Can you work these out from the drawing? Everything is in mm from the part's minimum corner. A direction names the side the tool comes from. Round coordinates to 2 decimals unless told otherwise and drop trailing zeros. Write each loop counter-clockwise with the first axis right and the second up, starting at its lowest first coordinate (ties: lowest second). Pieces come first, ordered by that corner, then holes. Notation, with made-up numbers: (-27.75, -34.5) - (-12.75, -34.5) arc R35 ccw to (-12.75, 1.5) - close; hole circle Ø2 at (21.5, 61). An arc over 180 degrees is marked (long way). Write each question's results on one line, items separated by ' | '. Start each with the question number.
(1) Please list where these lines run through material, in increasing order: line 1 (Z direction, x = 1.75, y = 4.25); line 2 (X direction, y = 4.25, z = 1.25); line 3 (Y direction, x = 19, z = 19). Write a range as [from, to].
(2) Imagine slicing it at B-B on x = 11.25. Write out the boundary of the cut face in (y, z), then the cut area to 3 significant figures.
(3) Imagine slicing it at A-A on y = 7. Write out the boundary of the cut face in (x, z) (1 decimal).
(4) Imagine slicing it at C-C on z = 12.5. Write out the boundary of the cut face in (x, y).
(5) For P1, Ø4, axis at y = 9, z = 11, coming from the -X side; P2, Ø5, axis at x = 2.5, z = 19, coming from the -Y side; P3, Ø0.9, axis at x = 14.5, z = 24, coming from the +Y side; P4, Ø9.5, axis at x = 12.5, z = 11, coming from the +Y side, each with a flat end and sliding along its axis, tell me the tip position at first contact or that it passes through.
(6) On a 3-axis mill with a long thin cutter (end or side, diameter ignored), from which of +Z, -Z, +X, -X, +Y, -Y can I reach the whole of each face in a straight line? I mean the marked faces 1, 2 and 3. Say none if no direction works.
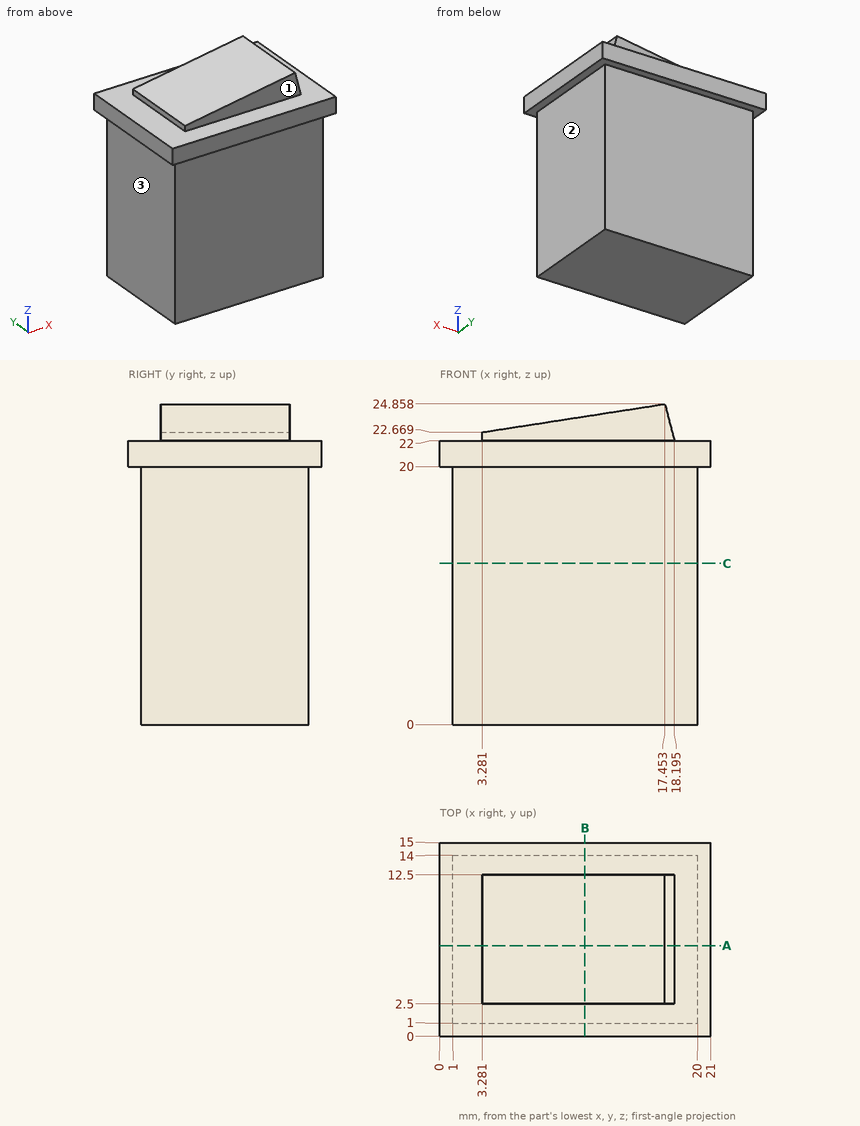
Response:
1) line 1: [0, 22] | line 2: [1, 20] | line 3: [1, 14]
2) outline: (0, 20) - (1, 20) - (1, 0) - (14, 0) - (14, 20) - (15, 20) - (15, 22) - (12.5, 22) - (12.5, 23.9) - (2.5, 23.9) - (2.5, 22) - (0, 22) - close | area: 309 mm²
3) outline: (0, 20) - (1, 20) - (1, 0) - (20, 0) - (20, 20) - (21, 20) - (21, 22) - (18.2, 22) - (17.5, 24.9) - (3.3, 22.7) - (3.3, 22) - (0, 22) - close
4) outline: (1, 1) - (20, 1) - (20, 14) - (1, 14) - close
5) P1: x = 1 | P2: y = 0 | P3: y = 12.5 | P4: y = 14
6) face 1: +Z, +X, -X, -Y | face 2: -Z, +X, +Y, -Y | face 3: -Z, -X, +Y, -Y
